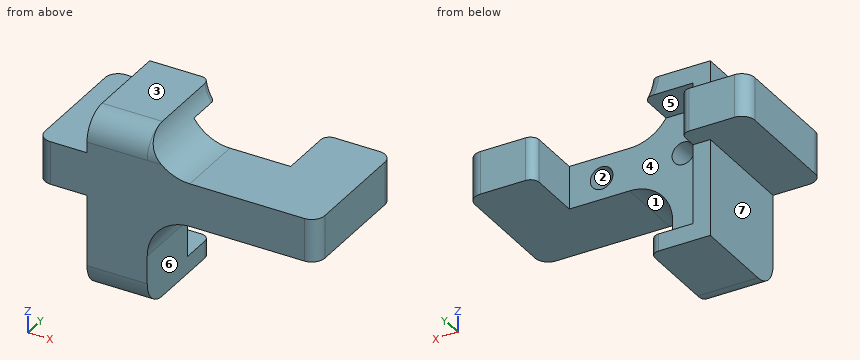
from build123d import *

# Parameters (mm, degrees)
SKETCH1_W           = 65
SKETCH1_H           = 30
BOSS_EXTRUDE1_DEPTH = 10
SKETCH2_W           = 34
SKETCH2_H           = 10
CUT_EXTRUDE1_DEPTH  = 14
SKETCH4_R           = 2.625
CUT_EXTRUDE3_DEPTH  = 45
FILLET1_R           = 3
SKETCH5_W           = 10
SKETCH5_H           = 4.5
SKETCH5_H_2         = 18.5
BOSS_EXTRUDE2_DEPTH = 16
CUT_EXTRUDE2_DEPTH  = 10
SKETCH6_W           = 10
SKETCH6_H           = 25
BOSS_EXTRUDE3_DEPTH = 4
BOSS_EXTRUDE4_START = -33
SKETCH6_2_W         = 10
SKETCH6_2_H         = 25
BOSS_EXTRUDE4_DEPTH = 4
BOSS_EXTRUDE7_REACH = 84.498
SKETCH7_W           = 4
SKETCH7_H           = 25
FILLET2_R           = 6
FILLET4_START       = 2.3595
FILLET4_DEPTH       = 13.6405
FILLET4_2_DEPTH     = 2.8314
FILLET4_START_2     = 6.0000001
FILLET4_3_DEPTH     = 18.9999999
FILLET4_START_3     = 25.5
FILLET4_4_DEPTH     = 9.886859967
FILLET4_5_DEPTH     = 6.00000009
FILLET7_R           = 2
BOSS_EXTRUDE8_DEPTH = 4.75


with BuildPart() as part:
    # Sketch1 → Boss-Extrude1 (new body)
    with BuildSketch(Plane.XY):
        with Locations((32.5, 15)):
            Rectangle(SKETCH1_W, SKETCH1_H)
    extrude(amount=BOSS_EXTRUDE1_DEPTH)

    # Sketch2 → Cut-Extrude1 (cut)
    with BuildSketch(Plane(origin=(0, 30, 0), x_dir=(1, 0, 0), z_dir=(0, 1, 0))):
        with Locations((32.5, -5)):
            Rectangle(SKETCH2_W, SKETCH2_H)
    extrude(amount=-CUT_EXTRUDE1_DEPTH, mode=Mode.SUBTRACT)

    # Sketch4 → Cut-Extrude3 (cut)
    with BuildSketch(Plane(origin=(0, 16, 0), x_dir=(1, 0, 0), z_dir=(0, 1, 0))):
        with Locations(Location((23, -5, 0), (0, 0, 270))):
            Circle(SKETCH4_R)
        with Locations(Location((42, -5, 0), (0, 0, 270))):
            Circle(SKETCH4_R)
    extrude(amount=-CUT_EXTRUDE3_DEPTH, mode=Mode.SUBTRACT)

    # Fillet1
    fillet1_edges = [part.edges().sort_by_distance(p)[0] for p in [
        (0, 30, 5),
        (0, 0, 5),
        (65, 0, 5),
        (65, 30, 5),
    ]]
    fillet(fillet1_edges, radius=FILLET1_R)

    # Sketch5 → Boss-Extrude2 (add)
    with BuildSketch(Plane(origin=(0, 16, 0), x_dir=(1, 0, 0), z_dir=(0, 1, 0))):
        with Locations((20.5, -12.25)):
            Rectangle(SKETCH5_W, SKETCH5_H)
        with BuildLine():
            Line((25.5, 0), (15.5, 0))
            Line((15.5, 0), (15.5, -10))
            Line((15.5, -10), (25.5, -10))
            Line((25.5, -10), (25.5, -5.80039053))
            ThreePointArc((25.5, -5.80039053), (20.375, -5), (25.5, -4.19960947))
            Line((25.5, -4.19960947), (25.5, 0))
        make_face()
        with Locations((20.5, 9.25)):
            Rectangle(SKETCH5_W, SKETCH5_H_2)
    extrude(amount=-BOSS_EXTRUDE2_DEPTH)

    # Sketch3 → Cut-Extrude2 (cut)
    with BuildSketch(Plane.XZ):
        Polygon((20.61843014, 9.125), (18.236860279, 5), (20.61843014, 0.875), (25.38156986, 0.875), (27.763139721, 5), (25.38156986, 9.125), align=None)
        Polygon((46.763139721, 5), (44.38156986, 9.125), (39.61843014, 9.125), (37.236860279, 5), (39.61843014, 0.875), (44.38156986, 0.875), align=None)
    extrude(amount=-CUT_EXTRUDE2_DEPTH, mode=Mode.SUBTRACT)

    # Sketch6 → Boss-Extrude3 (add)
    with BuildSketch(Plane.XY.offset(14.5)):
        with Locations((20.5, 12.5)):
            Rectangle(SKETCH6_W, SKETCH6_H)
    extrude(amount=BOSS_EXTRUDE3_DEPTH)

    # Sketch6<2> → Boss-Extrude4 (add)
    with BuildSketch(Plane.XY.offset(14.5).offset(BOSS_EXTRUDE4_START)):
        with Locations((20.5, 12.5)):
            Rectangle(SKETCH6_2_W, SKETCH6_2_H)
    extrude(amount=-BOSS_EXTRUDE4_DEPTH)

    # Boss-Extrude7: up to this face of the body (flat: up to its plane)
    boss_extrude7_end = Plane(part.part.faces().sort_by_distance((20.5, 12.5, -22.5))[0])
    # Sketch7 → Boss-Extrude7 (add, up to the picked face)
    with BuildSketch(Plane.XY.offset(18.5), mode=Mode.PRIVATE) as boss_extrude7_sk1:
        with Locations((13.5, 12.5)):
            Rectangle(SKETCH7_W, SKETCH7_H)
    boss_extrude7_tool1 = split(extrude(boss_extrude7_sk1.sketch, amount=-BOSS_EXTRUDE7_REACH, mode=Mode.PRIVATE), bisect_by=boss_extrude7_end, keep=Keep.BOTH, mode=Mode.PRIVATE)
    add(boss_extrude7_tool1.solids().sort_by(Axis((13.5, 12.5, 18.5), (0, 0, -1)))[0])

    # Fillet2
    fillet2_edges = [part.edges().sort_by_distance(p)[0] for p in [
        (18.5, 0, 18.5),
        (18.5, 0, -22.5),
    ]]
    fillet(fillet2_edges, radius=FILLET2_R)

    # Fillet4: read off the stored shape, not the designer's step
    # Fillet4 outline → Fillet4 (add)
    with BuildSketch(Plane(origin=(0, 0, 0), x_dir=(1, 0, 0), z_dir=(0, 1, 0)).offset(FILLET4_START)):
        with BuildLine():
            Line((25.5, -14.5), (27.035213422, -14.5))
            ThreePointArc((27.035213422, -14.5), (30.643443476, -11.196591569), (35.386859967, -10))
            Line((35.386859967, -10), (25.5, -10))
            Line((25.5, -10), (25.5, -14.5))
        make_face()
        with BuildLine():
            ThreePointArc((35.5, 0), (28.428932188, 2.928932188), (25.5, 10))
            Line((25.5, 10), (25.5, 0))
            Line((25.5, 0), (35.5, 0))
        make_face()
    extrude(amount=FILLET4_DEPTH)

    # Fillet4 2 outline → Fillet4 2 (add)
    with BuildSketch(Plane(origin=(0, 0, 0), x_dir=(1, 0, 0), z_dir=(0, 1, 0))):
        with BuildLine():
            ThreePointArc((35.5, 0), (28.428932188, 2.928932188), (25.5, 10))
            Line((25.5, 10), (25.5, 0))
            Line((25.5, 0), (35.5, 0))
        make_face()
    extrude(amount=FILLET4_2_DEPTH)

    # Fillet4 3 outline → Fillet4 3 (add)
    with BuildSketch(Plane(origin=(0, 0, 0), x_dir=(1, 0, 0), z_dir=(0, 1, 0)).offset(FILLET4_START_2)):
        with BuildLine():
            ThreePointArc((25.5, -18.5), (26.050866182, -16.416814258), (27.035213422, -14.5))
            Line((27.035213422, -14.5), (25.5, -14.5))
            Line((25.5, -14.5), (25.5, -18.5))
        make_face()
    extrude(amount=FILLET4_3_DEPTH)

    # Fillet4 4 outline → Fillet4 4 (add)
    with BuildSketch(Plane.YZ.offset(FILLET4_START_3)):
        with BuildLine():
            Line((0, 12.5), (0, 10))
            Line((0, 10), (2.3595, 10))
            Line((2.3595, 10), (2.3595, 14.5))
            Line((2.3595, 14.5), (6.0000001, 14.5))
            Line((6.0000001, 14.5), (6, 18.5))
            ThreePointArc((6, 18.5), (1.757359313, 16.742640687), (0, 12.5))
        make_face()
    extrude(amount=FILLET4_4_DEPTH)

    # Fillet4 5 outline → Fillet4 5 (cut)
    with BuildSketch(Plane(origin=(0, 0, 0), x_dir=(1, 0, 0), z_dir=(0, 1, 0))):
        with BuildLine():
            Line((25.5, -18.5), (25.272425218, -20))
            Line((25.272425218, -20), (35.386859967, -20))
            Line((35.386859967, -20), (35.386859967, -10))
            ThreePointArc((35.386859967, -10), (28.867657561, -12.417124556), (25.5, -18.5))
        make_face()
    extrude(amount=FILLET4_5_DEPTH, mode=Mode.SUBTRACT)

    # Fillet7
    fillet7_edges = [part.edges().sort_by_distance(p)[0] for p in [
        (25.5, 25, -20.5),
        (15.5, 30, 5),
        (49.5, 30, 5),
        (26.050866182, 25, 16.416814258),
    ]]
    fillet(fillet7_edges, radius=FILLET7_R)

    # Sketch3<2> → Boss-Extrude8 (add)
    with BuildSketch(Plane.XZ):
        Polygon((20.61843014, 9.125), (18.236860279, 5), (20.61843014, 0.875), (25.38156986, 0.875), (27.763139721, 5), (25.38156986, 9.125), align=None)
        Polygon((46.763139721, 5), (44.38156986, 9.125), (39.61843014, 9.125), (37.236860279, 5), (39.61843014, 0.875), (44.38156986, 0.875), align=None)
    extrude(amount=-BOSS_EXTRUDE8_DEPTH)


solid = part.part
Design review of the part built by this model. Coordinates are the model's own, in mm. Face numbers are marked on the shaded views. A direction names the side the tool comes from. Coordinates: 2 decimals unless noted, no trailing zeros. Loops run counter-clockwise (first coordinate to the right, second up) from the corner with the lowest first, then second, coordinate; pieces in that order, holes last.
Item 1: For the marked faces 5, 6 and 7, list the 3-axis set-ups (+Z, -Z, +X, -X, +Y, -Y) from which the entire face can be reached by the end or side of a thin tool; tool diameter is ignored.
Completed:
face 5: +X, +Y
face 6: -Z, +X, +Y, -Y
face 7: -Z, -X, +Y, -Y
Item 2: Add section C-C (y = 14). Write out the cut boundary in (x, z) (3 decimals).
Completed:
outline: (0, 0) - (11.5, 0) - (11.5, -22.5) - (25.5, -22.5) - (25.5, -10) arc R10 cw to (35.5, 0) - (65, 0) - (65, 10) - (35.387, 10) arc R10 cw to (25.5, 18.5) - (11.5, 18.5) - (11.5, 10) - (0, 10) - close; hole circle Ø5.25 at (23, 5); hole circle Ø5.25 at (42, 5)
Item 3: Draft analysis for pull direction X (two halves, no side actions). For the marked faces 1, 2, 3 and 4, state which applies: pulls with the +X half, pulls with the -X half, needs draft (parallel to the pull), parting line crosses it, or undercut.
Completed:
face 1: pulls with the +X half
face 2: undercut
face 3: needs draft
face 4: undercut
Item 4: Add section B-B (x = 42). Write out the cut boundary in (y, z) (3 decimals).
Completed:
outline: (0, 0) - (16, 0) - (16, 2.375) - (10, 2.375) - (10, 0.875) - (4.75, 0.875) - (4.75, 9.125) - (10, 9.125) - (10, 7.625) - (16, 7.625) - (16, 10) - (0, 10) - close
Item 5: Clearance check with flat-ended pins moving along their axes: pin 1 (6 mm diameter, centred on y = 12, z = 14, fed in from +X); pin 2 (4 mm diameter, centred on x = 22.5, z = 3, fed in from +Y); pin 3 (4 mm diameter, centred on x = 16, z = 15.5, fed in from +Y); pin 4 (10 mm diameter, centred on x = 32.5, z = -9, fed in from +Y). State where each tip first meets the part, or that it passes through.
Completed:
pin 1: stops at x = 31.03
pin 2: stops at y = 16
pin 3: stops at y = 25
pin 4: passes through
Item 6: Wall thickness on L1, parallel to X at y = 14.7, z = 5 (3 decimals); L2, parallel to X at y = 19.5, z = 8.5; L3, parallel to Z at x = 41, y = 8.5 (3 decimals): over which ranges is each line inside the solid? List them lowest first.
Completed:
L1: x = 0 to 20.375, 25.625 to 39.375, 44.625 to 65
L2: x = 0 to 15.5, 49.5 to 65
L3: z = 0 to 0.875, 9.125 to 10
Item 7: Add section D-D (z = -4). Write out the cut boundary in (x, y).
Completed:
outline: (11.5, 0) - (27.5, 0) - (27.5, 16) - (15.5, 16) - (15.5, 25) - (11.5, 25) - close
Item 8: Add section A-A (y = 19.5). Write out the cut boundary in (x, z).
Completed:
outline: (0, 0) - (11.5, 0) - (11.5, -22.5) - (25.5, -22.5) - (25.5, -18.5) - (15.5, -18.5) - (15.5, 14.5) - (27.04, 14.5) arc R10 cw to (25.5, 18.5) - (11.5, 18.5) - (11.5, 10) - (0, 10) - close; (49.5, 0) - (65, 0) - (65, 10) - (49.5, 10) - close
